```python
from build123d import *

# Parameters (mm, degrees)
F1_DEPTH = 152.4
F2_R     = 15.875
F3_DEPTH = 25.4
F4_R     = 7.9375
F5_DEPTH = 82.55


with BuildPart() as f1:
    # F0 (on Top) → F1 (new body)
    with BuildSketch(Plane.XY):
        Polygon((0, 79.375), (50.8, 79.375), (50.8, 80.9625), (-1.5875, 80.9625), (-1.5875, -1.5875), (50.8, -1.5875), (50.8, 0), (0, 0), align=None)
    extrude(amount=F1_DEPTH)

    # F2 (on face) → F3 (cut)
    with BuildSketch(Plane(origin=(-1.5875, 0, 0), x_dir=(0, -1, 0), z_dir=(-1, 0, 0))):
        with Locations((-39.6875, 76.2)):
            Circle(F2_R)
    extrude(amount=-F3_DEPTH, mode=Mode.SUBTRACT)

    # F4 (on face) → F5 (cut, through all)
    with BuildSketch(Plane.XZ.offset(1.5875)):
        with Locations((25.4, 31.75)):
            Circle(F4_R)
    extrude(amount=-F5_DEPTH, mode=Mode.SUBTRACT)


solid = f1.part
```
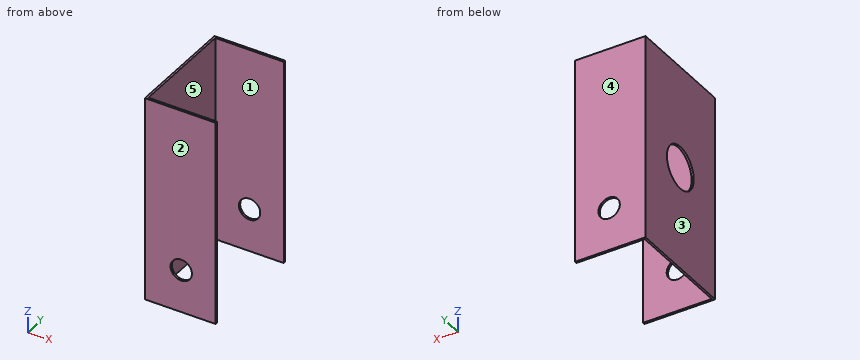
Could you check a few things on this model? Use its own coordinates, in mm. Face numbers are marked on the shaded views. A direction names the side the tool comes from. Round coordinates to 2 decimals unless told otherwise and drop trailing zeros. Loops run counter-clockwise (first coordinate to the right, second up) from the corner with the lowest first, then second, coordinate; pieces in that order, holes last. Notation, with made-up numbers: M -24.5,51 L 7.5,51 A24 ccw 7.5,87 Z; hole C 48,-36.5 d1. An arc over 180 degrees is marked long. Put each result on its own line as item: value.
Q1. Imagine slicing it at C-C (z = 76.2). Write out the boundary of the cut face in (x, y) (1 decimal), then the cut area to 3 significant figures.
Check result:
outline: M -1.6,-1.6 L 50.8,-1.6 L 50.8,0 L 0,0 L 0,23.8 L -1.6,23.8 Z; M -1.6,55.6 L 0,55.6 L 0,79.4 L 50.8,79.4 L 50.8,81 L -1.6,81 Z
area: 242 mm2
Q2. Imagine slicing it at D-D (x = 25.4). Write out the boundary of the cut face in (y, z) (1 decimal), then the cut area to 3 significant figures.
Check result:
outline: M -1.6,0 L 0,0 L 0,23.8 L -1.6,23.8 Z; M -1.6,39.7 L 0,39.7 L 0,152.4 L -1.6,152.4 Z; M 79.4,0 L 81,0 L 81,23.8 L 79.4,23.8 Z; M 79.4,39.7 L 81,39.7 L 81,152.4 L 79.4,152.4 Z
area: 433 mm2
Q3. On a 3-axis mill with a long thin cutter (end or side, diameter ignored), from which of +Z, -Z, +X, -X, +Y, -Y can I reach the whole of each face in a straight line? I mean the marked faces 1 and 2. Say none if no direction works.
Check result:
face 1: +Z, -Z, +X
face 2: +Z, -Z, +X, -X, -Y
Q4. Imagine slicing it at B-B (z = 31.75). Write out the boundary of the cut face in (x, y) (1 decimal), then the cut area to 3 significant figures.
Check result:
outline: M -1.6,-1.6 L 17.5,-1.6 L 17.5,0 L 0,0 L 0,79.4 L 17.5,79.4 L 17.5,81 L -1.6,81 Z; M 33.3,-1.6 L 50.8,-1.6 L 50.8,0 L 33.3,0 Z; M 33.3,79.4 L 50.8,79.4 L 50.8,81 L 33.3,81 Z
area: 242 mm2
Q5. I need wall thicknesses on probe 1 along Y at (x, z) = (4.5, 122.5) (1 decimal); probe 2 along Z at (x, y) = (25, 80); probe 3 along X at (y, z) = (43, 19). Which ranges of each line are inside material? Lowest first, please.
Check result:
probe 1: -1.6 to 0, 79.4 to 81
probe 2: 0 to 23.82, 39.68 to 152.4
probe 3: -1.59 to 0
Q6. Imagine slicing it at A-A (x = 42). Write out the boundary of the cut face in (y, z) (1 decimal), then the cut area to 3 significant figures.
Check result:
outline: M -1.6,0 L 0,0 L 0,152.4 L -1.6,152.4 Z; M 79.4,0 L 81,0 L 81,152.4 L 79.4,152.4 Z
area: 484 mm2
Q7. For pin 1 (14.5 mm diameter, centred on x = 25.4, z = 31.75, fed in from +Y); pin 2 (18.5 mm diameter, centred on x = 25.4, z = 31.75, fed in from +Y); pin 3 (12 mm diameter, centred on y = 71.5, z = 105.5, fed in from +X), each with a flat end and sliding along its axis, tell me the tip position at first contact or that it passes through.
Check result:
pin 1: through
pin 2: y = 80.96
pin 3: x = 0
Q8. Thinking about a two-plate mould opening in Y: for the marked faces 3, 4 and 5, which applies, released by +Y, released by -Y, zero draft, split by the parting line, or undercut?
Check result:
face 3: zero draft
face 4: released by +Y
face 5: undercut
